Input: part model. Units: mm. Frame: model coordinates. A direction names the side the tool comes from. Coordinates: 2 decimals unless noted, no trailing zeros. Order: outer loops, then holes, each group sorted by start corner. A loop starts at its lowest first (then second) coordinate and runs counter-clockwise, first axis right, second up. Notation, with made-up numbers: (84.25, 17) -> (132.25, 17) arc R23 ccw to (132.25, 34) -> close; hole circle Ø8 at (-36.5, 16.25). An arc over 180 degrees is marked (long way). Use one line per item in the form item = value. Start each with the question number.
1) Pin query (flat end, axial travel): pin 1 (2 mm diameter, centred on x = 30, y = 9.5, fed in from +Z); pin 2 (4 mm diameter, centred on x = 68.5, y = -3, fed in from -Z); pin 3 (2 mm diameter, centred on x = 69.5, z = 11.5, fed in from -Y). Return the tip coordinate at first contact, or that it passes through.
2) Draft query along Z for faces 4 (the flat face through (14.03, -9.52, -4.27)), 5 (the cylindrical face through (33.97, -0.77, 5.87)), 6 (the flat face through (24, -6, 3)). Return one class per face: pulls with the +Z half, pulls with the -Z half, needs draft (parallel to the pull), parting line crosses it, or undercut.
3) Section query A-A on x = -33. Output: boundary loops of the cut face in (y, z), then the cut area to 3 significant figures.
4) Access query for faces 1 (the cylindrical face through (21.97, 6.26, 12.43)), 2 (the flat face through (22.03, 4.27, -9.52)), 3 (the cylindrical face through (-6.03, -0.77, 5.87)). Directions: +Z, -Z, +X, -X, +Y, -Y. A direction counts if a zero-diameter tool reaches every point of the face in a straight line with its end or side. Return the directions, or none.
5) Ray query, line 1 along X through (y, z) = (1, -2.25); line 2 along Y through (x, z) = (10.5, 2); line 3 along Y through (x, z) = (-35, 4.25). Return the intervals inside material, ascending.
from build123d import *

# Parameters (mm, degrees)
F3_DEPTH = 25
F4_DEPTH = 250
F5_DEPTH = 22.8


with BuildPart() as f1:
    # F0 (on Top) → F1 (revolve)
    with BuildSketch(Plane.XY):
        Polygon((-41, 5.919), (-41, 0), (85, 0), (85, 5.911648), (72, 5.911648), (72, 13.919), (68, 13.919), (68, 5.919), (64, 5.919), (64, 13.919), (60, 13.919), (60, 5.919), (56, 5.919), (56, 13.919), (52, 13.919), (52, 5.919), (48, 5.919), (48, 13.919), (44, 13.919), (44, 5.919), (40, 5.919), (40, 13.919), (36, 13.919), (36, 5.919), (32, 5.919), (32, 13.919), (28, 13.919), (28, 5.919), (24, 5.919), (24, 13.919), (20, 13.919), (20, 5.919), (16, 5.919), (16, 13.919), (12, 13.919), (12, 5.919), (8, 5.919), (8, 13.919), (4, 13.919), (4, 5.919), (0, 5.919), (0, 13.919), (-4, 13.919), (-4, 5.919), (-8, 5.919), (-8, 13.919), (-12, 13.919), (-12, 5.919), (-16, 5.919), (-16, 13.919), (-20, 13.919), (-20, 5.919), (-24, 5.919001), (-24, 13.919), (-28, 13.919), (-28, 5.919), align=None)
    revolve(axis=Axis((22, 0, 0), (1, 0, 0)))

    # F2 (on face) → F3 (cut)
    with BuildSketch(Plane.YZ.offset(72)):
        Polygon((-2.309401, -4), (2.309401, -4), (4.618802, 0), (2.309401, 4), (-2.309401, 4), (-4.618802, 0), align=None)
    extrude(amount=F3_DEPTH, mode=Mode.SUBTRACT)

    # F2 (on face) → F4 (cut)
    with BuildSketch(Plane.YZ.offset(72)):
        with BuildLine():
            Line((0, 7.919), (0, 13.919))
            ThreePointArc((0, 13.919), (-4.446775, 13.18957), (-8.42748, 11.077732))
            Line((-8.42748, 11.077732), (0, 7.919))
        make_face()
        with BuildLine():
            ThreePointArc((13.919, 0), (13.18957, 4.446775), (11.077732, 8.42748))
            Line((11.077732, 8.42748), (7.919, 0))
            Line((7.919, 0), (13.919, 0))
        make_face()
        with BuildLine():
            ThreePointArc((0, -13.919), (4.446775, -13.18957), (8.42748, -11.077732))
            Line((8.42748, -11.077732), (0, -7.919))
            Line((0, -7.919), (0, -13.919))
        make_face()
        with BuildLine():
            Line((-7.919, 0), (-13.919, 0))
            ThreePointArc((-13.919, 0), (-13.18957, -4.446775), (-11.077732, -8.42748))
            Line((-11.077732, -8.42748), (-7.919, 0))
        make_face()
    extrude(amount=-F4_DEPTH, mode=Mode.SUBTRACT)

    # F2 (on face) → F5 (cut)
    with BuildSketch(Plane.YZ.offset(72)):
        Polygon((-2.309401, -4), (2.309401, -4), (4.618802, 0), (2.309401, 4), (-2.309401, 4), (-4.618802, 0), align=None)
    extrude(amount=F5_DEPTH, mode=Mode.SUBTRACT)


solid = f1.part
Answers below:
q1.pin_1 = 11.02
q1.pin_2 = -13.88
q1.pin_3 = -9.14
q2.face_4 = undercut
q2.face_5 = parting line crosses it
q2.face_6 = needs draft
q3.outline = circle Ø11.84 at (0, 0)
q3.area = 110 mm^2
q4.face_1 = +Z, +X, -X, +Y
q4.face_2 = -Z, +X, -X
q4.face_3 = none
q5.line_1 = -41 to 72
q5.line_2 = -5.57 to 5.57
q5.line_3 = -4.12 to 4.12
